For this review, take the finished solid that the model builds, in its own axes (mm). Face numbers are marked on the shaded views. A direction names the side the tool comes from. Coordinates: 2 decimals unless noted, no trailing zeros. Loops run counter-clockwise (first coordinate to the right, second up) from the corner with the lowest first, then second, coordinate; pieces in that order, holes last. Notation, with made-up numbers: (-24, 29.25) - (-11, 29.25) arc R9 ccw to (-11, 37.25) - close; hole circle Ø7 at (-12.5, 81.5). An arc over 180 degrees is marked (long way). Answer as a JSON object with one key per item and string values. Group by question number.
Item 1: Clearance check with flat-ended pins moving along their axes: pin 1 (4 mm diameter, centred on y = 34.5, z = -36, fed in from -X); pin 2 (6 mm diameter, centred on x = 19, z = -14.5, fed in from +Y); pin 3 (4 mm diameter, centred on x = 56, y = 16, fed in from -Z). State where each tip first meets the part, or that it passes through.
Item 2: Tool access review of the marked faces 1, 2 and 3: name each direction out of +Z, -Z, +X, -X, +Y, -Y from which nothing blocks a thin tool from reaching the whole face with its end or side.
Item 3: We need section D-D (x = 45). Give the boundary of the cut face in (y, z), then the cut area to 3 significant figures.
Item 4: We need section A-A (z = -28.5). Give the boundary of the cut face in (x, y), then the cut area to 3 significant figures.
Item 5: To check wall thickness, follow line 1 (Y direction, x = 18, z = -6); line 2 (Z direction, x = 11, y = 22); line 3 (Y direction, x = 55, z = -32.5). State the ranges of each line that lie inside material, in increasing order.
Item 6: We need section C-C (y = 29). Give the boundary of the cut face in (x, z), then the cut area to 3 significant figures.
Item 7: We need section B-B (x = 33). Give the boundary of the cut face in (y, z).
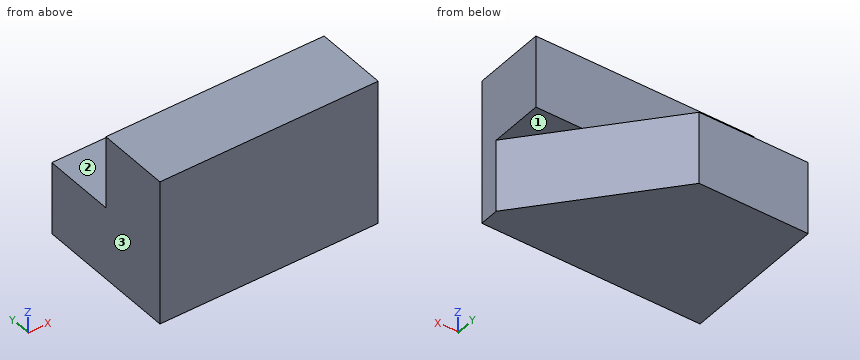
Autodesk Inventor part; units mm, degrees
ref_plane "YZ Plane" through (0, 0, 0) normal (1, 0, 0) x (0, 1, 0)
ref_plane "XZ Plane" through (0, 0, 0) normal (0, 1, 0) x (-1, 0, 0)
ref_plane "XY Plane" through (0, 0, 0) normal (0, 0, 1) x (1, 0, 0)
sketch "草圖1" plane through (0, 0, 0) normal (1, 0, 0) x (0, 1, 0)
  line L0 (0, 0) -> (20, 0)
  line L1 (20, 0) -> (20, -20)
  line L2 (20, -20) -> (0, -20)
  line L3 (0, -20) -> (0, 0)
  line L4 (0, 0) -> (5.3281, 0)
  line L5 (5.3281, 0) -> (5.3281, -40)
  line L6 (5.3281, -40) -> (0, -40)
  line L7 (0, -40) -> (0, 0)
  dimension "d0" = 40
  dimension "d1" = 20
  dimension "d2" = 20
extrude "擠出1" add sketch "草圖1" along normal blind 60
sketch "草圖2" plane through (0, 0, -40) normal (0, 0, -1) x (-1, 0, 0)
  line L0 (0, 0) -> (0, 5.3281)
  line L1 (0, 0) -> (0, 40)
  line L2 (0, 40) -> (-30, 40)
  line L3 (0, 5.3281) -> (-60, 5.3281)
  line L4 (-30, 40) -> (-60, 5.3281)
  line L5 (-60, 5.3281) -> (-60, 0)
  line L6 (0, 0) -> (-60, 0)
  line L7 (-60, 0) -> (0, 0)
  dimension "d5" = 30
  dimension "d6" = 40
extrude "擠出2" add sketch "草圖2" against normal up to surface (20 mm away) contours L3 L4 L2 L1
properties part number "41 (61598.433 mm^3)"
Check sheet entries:
{
 "1": {"pin 1": "stops at x = 0", "pin 2": "stops at y = 20", "pin 3": "stops at z = -20"},
 "2": {"face 1": "-Z, +X, +Y", "face 2": "+Z, +X, -X, +Y", "face 3": "+Z, -Z, -X, +Y, -Y"},
 "3": {"outline": "(0, -40) - (22.66, -40) - (22.66, -20) - (20, -20) - (20, 0) - (0, 0) - close", "area": "853 mm2"},
 "4": {"outline": "(0, 0) - (60, 0) - (60, 5.33) - (30, 40) - (0, 40) - close", "area": "1,880 mm2"},
 "5": {"line 1": "y = 0 to 20", "line 2": "z = -40 to -20", "line 3": "y = 0 to 11.11"},
 "6": {"outline": "(0, -40) - (39.52, -40) - (39.52, -20) - (0, -20) - close", "area": "790 mm2"},
 "7": {"outline": "(0, -40) - (36.53, -40) - (36.53, -20) - (20, -20) - (20, 0) - (0, 0) - close"}
}
